CAD build for the part. Positions are in the model's coordinates, mm. Round coordinates to 2 decimals unless told otherwise and drop trailing zeros. Order: outer loops, then holes, each group sorted by start corner. A loop starts at its lowest first (then second) coordinate and runs counter-clockwise, first axis right, second up.
```python
from build123d import *

# Parameters (mm, degrees)
SKETCH012_W     = 4.485072
SKETCH012_H     = 0.815651
POCKET003_DEPTH = 8.001
CHAMFER003_SIZE = 0.15


with BuildPart() as part:
    # Sketch011 → Revolution001 (revolve)
    with BuildSketch(Plane.XZ):
        Polygon((-1.45, 0), (-1.45, 5), (-2.2, 8), (-2.45, 8), (-2.45, 0), align=None)
    revolve(axis=Axis((0, 0, 0), (0, 0, 1)))

    # Sketch012 (on Face5 of Revolution001) → Pocket003 (cut, through all)
    with BuildSketch(Plane(origin=(0, 0, 0), x_dir=(1, 0, 0), z_dir=(0, 0, -1))):
        with Locations((0.20817, 2.2078255)):
            Rectangle(SKETCH012_W, SKETCH012_H)
    extrude(amount=-POCKET003_DEPTH, mode=Mode.SUBTRACT)

    # Chamfer003
    chamfer003_edges = [part.edges().sort_by_distance(p)[0] for p in [
        (-2.244392, -0.982449, 0),
        (0, -1.8, 0),
        (0.982449, 2.244392, 0),
        (1.45, 0, 0),
    ]]
    chamfer(chamfer003_edges, length=CHAMFER003_SIZE)


solid = part.part
```
1. Cut at B-B, the plane x = 0. Write the cut outline in (y, z).
2. Cut at A-A, the plane y = 0. Write the cut outline in (x, z).
3. Mould opens along Y. For faces 1 (the face through (0, 2, 0)), 2 (the face through (1.45, -0.06, 2.61)), 3 (the face through (0.08, 2.45, 4.02)), 4 (the face through (0, -1.8, 4)) say: released by +Y, released by -Y, zero draft, split by the parting line, or undercut.
4. Drill centre lines: line 1 (X direction, y = 0, z = 3.5); line 2 (X direction, y = 0.25, z = 6.75); line 3 (Y direction, x = 1.4, z = 6.25). Where is each one in solid material? Low to high.
Outcome:
1. outline: (-1.8, 0.15) - (-1.65, 0) - (-1.6, 0) - (-1.45, 0.15) - (-1.45, 5) - (-1.8, 6.4) - close; (1.45, 0.15) - (1.6, 0) - (2.3, 0) - (2.45, 0.15) - (2.45, 8) - (2.2, 8) - (1.45, 5) - close
2. outline: (-2.45, 0.15) - (-2.3, 0) - (-1.6, 0) - (-1.45, 0.15) - (-1.45, 5) - (-2.2, 8) - (-2.45, 8) - close; (1.45, 0.15) - (1.6, 0) - (2.3, 0) - (2.45, 0.15) - (2.45, 8) - (2.2, 8) - (1.45, 5) - close
3. face 1: zero draft
3. face 2: undercut
3. face 3: split by the parting line
3. face 4: released by -Y
4. line 1: x = -2.45 to -1.45, 1.45 to 2.45
4. line 2: x = -2.44 to -1.87, 1.87 to 2.44
4. line 3: y = -1.8 to -1.07, 1.07 to 2.01
